Read the model definition and answer for the solid it produces. Units are mm, in the model's axes. A direction names the side the tool comes from. Coordinates: 2 decimals unless noted, no trailing zeros. Order: outer loops, then holes, each group sorted by start corner. A loop starts at its lowest first (then second) coordinate and runs counter-clockwise, first axis right, second up.
from build123d import *

# Parameters (mm, degrees)
SKETCH_1_R               = 12.4
SKETCH_1_R_2             = 1.5999999999999976
SKETCH_1_R_3             = 1.5999999999999506
SKETCH_1_R_4             = 1.6
EXTRUDE_1_DEPTH          = 20
EXTRUDE_START            = -9.5
SKETCH_2_R               = 12.4
EXTRUDE_2_DEPTH          = 9.5
SKETCH_4_R               = 2.999999999999999
SKETCH_4_R_2             = 3.0000000000000004
SKETCH_4_R_3             = 3
CUT_EXTRUDE_1_DEPTH      = 3.3
SKETCH_5_R               = 1.6
SKETCH_5_R_2             = 1.5999999999999956
SKETCH_5_R_3             = 1.6000000000000036
EXTRUDE_3_DEPTH          = 9
EXTRUDE_4_DEPTH          = 4
CUT_EXTRUDE_2_DEPTH      = 60.910683521388734
CUT_EXTRUDE_3_DEPTH      = 92.54938567789519
CUT_EXTRUDE_3_DEPTH_BACK = 3.3
SKETCH_8_R               = 2.9999999999999982
SKETCH_8_R_2             = 2.9999999999999973
CHAMFER_1_SIZE           = 5
EXTRUDE_7_REACH          = 87.92
SKETCH_9_R               = 18.6
CUT_EXTRUDE_7_DEPTH      = 67.95700121719909
EXTRUDE_START_2          = -5.7
SKETCH_18_R              = 2.999999999999999
SKETCH_18_R_2            = 1.6000000000000036
EXTRUDE_8_DEPTH          = 5.7
SKETCH_19_R              = 2.999999999999999
CUT_EXTRUDE_8_DEPTH      = 90.42136219796699
SKETCH_20_R              = 18.6
CUT_EXTRUDE_9_DEPTH      = 7
CUT_EXTRUDE_10_DEPTH     = 7
FILLET_2_R               = 2
SKETCH_22_R              = 12.600000000000001
CUT_EXTRUDE_11_DEPTH     = 7
FILLET_3_R               = 2
CUT_EXTRUDE_12_DEPTH     = 87.00937458341387
FILLET_4_R               = 3
CUT_EXTRUDE_13_DEPTH     = 60.91068362153782
FILLET_5_R               = 1
FILLET_6_R               = 5
CHAMFER_2_SIZE           = 1


with BuildPart() as part:
    # 草图1 → 凸台-拉伸1 (new body)
    with BuildSketch(Plane(origin=(0, 0, 0), x_dir=(1, 0, 0), z_dir=(0, 1, 0))):
        with Locations(Location((0, 0, 0), (0, 0, 270))):
            Circle(SKETCH_1_R)
        with Locations(Location((9.000000000000002, 2.1e-15, 0), (0, 0, 270))):
            Circle(SKETCH_1_R_2, mode=Mode.SUBTRACT)
        with Locations(Location((-4.500000000000038, -7.794228634059926, 0), (0, 0, 270))):
            Circle(SKETCH_1_R_3, mode=Mode.SUBTRACT)
        with Locations(Location((-4.499999999999964, 7.794228634060018, 0), (0, 0, 270))):
            Circle(SKETCH_1_R_4, mode=Mode.SUBTRACT)
    extrude(amount=EXTRUDE_1_DEPTH)

    # 草图2 → 凸台-拉伸2 (add)
    with BuildSketch(Plane(origin=(0, 20, 0), x_dir=(1, 0, 0), z_dir=(0, 1, 0)).offset(EXTRUDE_START)):
        with BuildLine():
            Line((0, 30), (25.15, 30))
            Line((25.15, 30), (25.15, -30))
            Line((25.15, -30), (0, -30))
            ThreePointArc((0, -30), (-30, 3.67e-15), (0, 30))
        make_face()
        with Locations(Location((0, 0, 0), (0, 0, 270))):
            Circle(SKETCH_2_R, mode=Mode.SUBTRACT)
    extrude(amount=EXTRUDE_2_DEPTH)

    # 草图4 → 切除-拉伸1 (cut)
    with BuildSketch(Plane(origin=(0, 20, 0), x_dir=(1, 0, 0), z_dir=(0, 1, 0))):
        with Locations(Location((9.000000000000002, 2.1e-15, 0), (0, 0, 270))):
            Circle(SKETCH_4_R)
        with Locations(Location((-4.499999999999964, 7.794228634060018, 0), (0, 0, 270))):
            Circle(SKETCH_4_R_2)
        with Locations(Location((-4.500000000000038, -7.794228634059926, 0), (0, 0, 270))):
            Circle(SKETCH_4_R_3)
    extrude(amount=-CUT_EXTRUDE_1_DEPTH, mode=Mode.SUBTRACT)

    # 草图5 → 凸台-拉伸3 (add)
    with BuildSketch(Plane(origin=(0, 0, -30), x_dir=(-1, 0, -1.7e-16), z_dir=(1.7e-16, 0, -1))):
        Polygon((-25.15, 20), (-25.15, 62.3), (-14.078932188134525, 62.3), (28.22106781186546, 20), align=None)
        with Locations((-15.500000000000005, 25.649999999999995)):
            Circle(SKETCH_5_R, mode=Mode.SUBTRACT)
        with Locations((-15.499999999999998, 56.64999999999999)):
            Circle(SKETCH_5_R_2, mode=Mode.SUBTRACT)
        with Locations((15.499999999999995, 25.64999999999999)):
            Circle(SKETCH_5_R_3, mode=Mode.SUBTRACT)
    extrude(amount=-EXTRUDE_3_DEPTH)

    # 草图6 → 凸台-拉伸4 (add)
    with BuildSketch(Plane(origin=(25.15, 0, 0), x_dir=(0, 0, -1), z_dir=(1, 0, 0))):
        Polygon((-24.999999999999996, 19.999999999999996), (20.999999999999996, 62.3), (20.999999999999996, 20), align=None)
    extrude(amount=-EXTRUDE_4_DEPTH)

    # 草图7 → 切除-拉伸2 (cut, through all)
    with BuildSketch(Plane.XZ.offset(-20)):
        with BuildLine():
            Line((-28.22106781186546, -30.000000000000004), (3.9e-15, -30))
            ThreePointArc((3.9e-15, -30), (-11.618950038622252, -27.65863337187866), (-21.42428528562855, -21))
            Line((-21.42428528562855, -21), (-28.22106781186546, -21.000000000000004))
            Line((-28.22106781186546, -21.000000000000004), (-28.22106781186546, -30.000000000000004))
        make_face()
    extrude(amount=-CUT_EXTRUDE_2_DEPTH, mode=Mode.SUBTRACT)

    # 草图8 → 切除-拉伸3 (cut, two sides: drawn at the far end of the back side and taken through both)
    with BuildSketch(Plane(origin=(0, 0, -30), x_dir=(-1, 0, -1.7e-16), z_dir=(1.7e-16, 0, -1)).offset(-CUT_EXTRUDE_3_DEPTH_BACK)):
        with Locations(Location((-15.499999999999998, 56.64999999999999, 0), (0, 0, 180))):
            Circle(SKETCH_8_R)
        with Locations(Location((-15.500000000000005, 25.649999999999995, 0), (0, 0, 180))):
            Circle(SKETCH_8_R_2)
    extrude(amount=CUT_EXTRUDE_3_DEPTH + CUT_EXTRUDE_3_DEPTH_BACK, mode=Mode.SUBTRACT)

    # 倒角1
    chamfer_1_edges = [part.edges().sort_by_distance(p)[0] for p in [
        (12.575, 20, 30),
        (-27.65863337187878, 20, 11.618950038621964),
    ]]
    chamfer(chamfer_1_edges, length=CHAMFER_1_SIZE)

    # 凸台-拉伸7: up to this face of the body (flat: up to its plane)
    extrude_7_end = Plane(part.part.faces().sort_by_distance((13.111797909, 34.333599445, -30))[0])
    # 草图9 → 凸台-拉伸7 (add, up to the picked face)
    with BuildSketch(Plane.XY.offset(-20.999999999999996), mode=Mode.PRIVATE) as extrude_7_sk1:
        with Locations((-1.73e-15, 41.14999999999999)):
            Circle(SKETCH_9_R)
    extrude_7_tool1 = split(extrude(extrude_7_sk1.sketch, amount=-EXTRUDE_7_REACH, mode=Mode.PRIVATE), bisect_by=extrude_7_end, keep=Keep.BOTH, mode=Mode.PRIVATE)
    add(extrude_7_tool1.solids().sort_by(Axis((0, 41.15, -21), (0, 0, -1)))[0])

    # 草图17 → 切除-拉伸7 (cut, through all)
    with BuildSketch(Plane.XZ.offset(-10.5)):
        with BuildLine():
            Line((0, -30), (-18.6, -30))
            Line((-18.6, -30), (-18.6, -23.538054295119636))
            ThreePointArc((-18.6, -23.538054295119636), (-9.845262087583318, -28.338504096490247), (0, -30))
        make_face()
    extrude(amount=-CUT_EXTRUDE_7_DEPTH, mode=Mode.SUBTRACT)

    # 草图18 → 凸台-拉伸8 (add)
    with BuildSketch(Plane.XY.offset(-20.999999999999996).offset(EXTRUDE_START_2)):
        with Locations((-15.5, 25.64999999999999)):
            Circle(SKETCH_18_R)
        with Locations(Location((-15.5, 25.64999999999999, 0), (0, 0, 180))):
            Circle(SKETCH_18_R_2, mode=Mode.SUBTRACT)
    extrude(amount=EXTRUDE_8_DEPTH)

    # 草图19 → 切除-拉伸8 (cut, through all)
    with BuildSketch(Plane(origin=(4.63e-15, 0, -26.7), x_dir=(-1, 0, -1.7e-16), z_dir=(1.7e-16, 0, -1))):
        with Locations((15.500000000000002, 25.64999999999999)):
            Circle(SKETCH_19_R)
    extrude(amount=CUT_EXTRUDE_8_DEPTH, mode=Mode.SUBTRACT)

    # 草图20 → 切除-拉伸9 (cut)
    with BuildSketch(Plane.XY.offset(-20.999999999999996)):
        with Locations((-1.73e-15, 41.14999999999999)):
            Circle(SKETCH_20_R)
    extrude(amount=-CUT_EXTRUDE_9_DEPTH, mode=Mode.SUBTRACT)

    # 草图21 → 切除-拉伸10 (cut)
    with BuildSketch(Plane.XY.offset(-27.999999999999996)):
        with BuildLine():
            Line((9.132536191757762, 57.353604003623225), (-10.770329614269013, 25.985567930186104))
            Line((-10.770329614269013, 25.985567930186104), (-10.770329614269013, 56.31443206981388))
            ThreePointArc((-10.770329614269013, 56.31443206981388), (-0.9698254485780136, 59.72469888313914), (9.132536191757762, 57.353604003623225))
        make_face()
    extrude(amount=-CUT_EXTRUDE_10_DEPTH, mode=Mode.SUBTRACT)

    # 圆角2
    fillet_2_edges = [part.edges().sort_by_distance(p)[0] for p in [
        (9.132536191757753, 57.353604003623225, -24.499999999999996),
        (-16.203604003623234, 32.01746380824223, -23.123818927861777),
    ]]
    fillet(fillet_2_edges, radius=FILLET_2_R)

    # 草图22 → 切除-拉伸11 (cut)
    with BuildSketch(Plane.XY.offset(-27.999999999999996)):
        with Locations((1e-15, 41.14999999999999)):
            Circle(SKETCH_22_R)
    extrude(amount=-CUT_EXTRUDE_11_DEPTH, mode=Mode.SUBTRACT)

    # 圆角3
    fillet_3_edges = [part.edges().sort_by_distance(p)[0] for p in [
        (5.91155300792769, 52.27715332124353, -29),
        (-7.549346430438945, 31.062018612565794, -28.51729458674393),
    ]]
    fillet(fillet_3_edges, radius=FILLET_3_R)

    # 草图23 → 切除-拉伸12 (cut, through all)
    with BuildSketch(Plane.ZY.offset(-21.15)):
        Polygon((-3.5400992489435197, 39.45183914325861), (-21.000000000000007, 55.50735657303446), (-21.000000000000004, 23.396321713482756), align=None)
        Polygon((17.613201001408648, 20), (0.1533002503521459, 36.05551742977586), (-17.306600500704334, 20), align=None)
    extrude(amount=-CUT_EXTRUDE_12_DEPTH, mode=Mode.SUBTRACT)

    # 圆角4
    fillet_4_edges = [part.edges().sort_by_distance(p)[0] for p in [
        (23.15, 20, -17.306600500704334),
        (23.15, 36.05551742977586, 0.15330025035214767),
        (23.15, 20, 17.613201001408648),
        (23.15, 23.396321713482756, -21.000000000000004),
        (23.15, 55.50735657303446, -21.000000000000007),
        (23.15, 39.45183914325861, -3.540099248943516),
    ]]
    fillet(fillet_4_edges, radius=FILLET_4_R)

    # 草图24 → 切除-拉伸13 (cut, through all)
    with BuildSketch(Plane(origin=(0, 20, 0), x_dir=(1, 0, 0), z_dir=(0, 1, 0))):
        with BuildLine():
            Line((25.15, -24.999999999999996), (25.15, -30))
            Line((25.15, -30), (20.15, -30))
            ThreePointArc((20.15, -30), (23.685533905932736, -28.535533905932734), (25.15, -24.999999999999996))
        make_face()
    extrude(amount=-CUT_EXTRUDE_13_DEPTH, mode=Mode.SUBTRACT)

    # 圆角5
    fillet_5_edges = [part.edges().sort_by_distance(p)[0] for p in [
        (-21.42428528562855, 20.898391263118448, -21.000000000000007),
    ]]
    fillet(fillet_5_edges, radius=FILLET_5_R)

    # 圆角6
    fillet_6_edges = [part.edges().sort_by_distance(p)[0] for p in [
        (25.15, 36.4, -29.999999999999996),
    ]]
    fillet(fillet_6_edges, radius=FILLET_6_R)

    # 倒角2
    chamfer_2_edges = [part.edges().sort_by_distance(p)[0] for p in [
        (3.8e-15, 0, -12.4),
    ]]
    chamfer(chamfer_2_edges, length=CHAMFER_2_SIZE)


solid = part.part
Q1. The part is cut by section C-C, the plane z = 0. Determine the outline of the cut face in (x, y), then the cut area to 3 significant figures.
Q2. Which of the six approach directions +Z, -Z, +X, -X, +Y, -Y give full straight-line access (tool end or side, diameter ignored) to faces 4 (the flat face through (21.15, 37, -5)), 5 (the cylindrical face through (10.294, 57.56, -24.451)), 6 (the cylindrical face through (-1.97, 18.37, 9.41)), 7 (the cylindrical face through (23.178, 27.504, -19.25))?
Q3. Each of these flat-tipped pins is pushed along its axis until it touches: P1, Ø3.5, axis at x = 15.5, y = 25.65, coming from the -Z side; P2, Ø1.5, axis at y = 40.5, z = 1, coming from the -X side; P3, Ø3, axis at x = 2.5, z = -21.5, coming from the +Y side. Where does it stop, or does it pass through?
Q4. The part is cut by section A-A, the plane y = 47. Determine the outline of the cut face in (x, z), then the cut area to 3 significant figures.
Q5. Determine the mould class of faces 1 (the flat face through (11.5, 35.5, -28)), 2 (the cylindrical face through (23.72, 36.76, -28.5)), 3 (the flat face through (-6, 16.7, 9)) for opening direction Y: +Y half, -Y half, draft (parallel to the pull), parting line (faces both ways), or undercut.
Q6. Straight lines are drawn through the part: L1, parallel to Y at x = 15.5, z = -27.7; L2, parallel to Z at x = -3.5, y = 16.5; L3, parallel to Y at x = 17, z = 2. For each, find the intervals that lie inside material, in ascending order.
Q7. The part is cut by section B-B, the plane x = 15.5. Determine the outline of the cut face in (y, z), then the cut area to 3 significant figures.
Q8. The part is cut by section D-D, the plane y = 38.5. Determine the outline of the cut face in (x, z), then the cut area to 3 significant figures.
Computed values:
1. outline: (-30, 10.5) - (-12.4, 10.5) - (-12.4, 1) - (-11.4, 0) - (7.4, 0) - (7.4, 16.7) - (6, 16.7) - (6, 20) - (-25, 20) - (-30, 15) - close; (10.6, 0) - (11.4, 0) - (12.4, 1) - (12.4, 10.5) - (25.15, 10.5) - (25.15, 20) - (12, 20) - (12, 16.7) - (10.6, 16.7) - close; (21.15, 34.98) - (25.15, 34.98) - (25.15, 42.99) - (21.15, 42.99) - close
1. area: 730 mm2
2. face 4: +Z, -X, +Y
2. face 5: +Z, -X
2. face 6: +Y
2. face 7: +X, -X
3. P1: stops at z = -26.7
3. P2: stops at x = 21.15
3. P3: stops at y = 22.99
4. outline: (11.16, -30) - (20.15, -30) arc R5 ccw to (25.15, -25) - (25.15, -21) - (17.66, -21) - (17.66, -28) - (11.16, -28) - close; (21.15, -11.75) - (25.15, -11.75) - (25.15, -4.36) - (21.15, -4.36) - close
4. area: 105 mm2
5. face 1: undercut
5. face 2: draft
5. face 3: +Y half
6. L1: y = 10.5 to 22.65, 28.65 to 30.87, 51.43 to 53.65, 59.65 to 62.3
6. L2: z = -29.8 to -9.04, -6.55 to 6.55, 9.04 to 28.28
6. L3: y = 10.5 to 20
7. outline: (10.5, -30) - (22.65, -30) - (22.65, -26.7) - (24.05, -26.7) - (24.05, -21) - (20, -21) - (20, 25) - (15, 30) - (10.5, 30) - close; (27.25, -26.7) - (28.65, -26.7) - (28.65, -30) - (53.65, -30) - (53.65, -26.7) - (55.05, -26.7) - (55.05, -21) - (51.43, -21) - (51.43, -28) - (30.87, -28) - (30.87, -21) - (27.25, -21) - close; (58.25, -26.7) - (59.65, -26.7) - (59.65, -30) - (62.3, -30) - (62.3, -21) - (58.25, -21) - close
7. area: 718 mm2
8. outline: (12.32, -30) - (20.15, -30) arc R5 ccw to (25.15, -25) - (25.15, -21) - (18.41, -21) - (18.41, -28) - (12.32, -28) - close; (21.15, -5.13) - (25.15, -5.13) - (25.15, 4.88) - (21.15, 4.88) - close
8. area: 108 mm2
